Here's how the part is built. I have some questions about the finished solid (model axes, mm). A direction names the side the tool comes from. Round coordinates to 2 decimals unless told otherwise and drop trailing zeros. Write each loop counter-clockwise with the first axis right and the second up, starting at its lowest first coordinate (ties: lowest second). Pieces come first, ordered by that corner, then holes. Notation, with made-up numbers: (34, 25.25) -> (65, 25.25) arc R9 cw to (65, 34.25) -> close; hole circle Ø11 at (-16.75, 64). An arc over 180 degrees is marked (long way). Answer as CSV lines item,"result".
```python
from build123d import *

# Parameters (mm, degrees)
FILLET1_R           = 0.25
SKETCH2_R           = 3
BOSS_EXTRUDE1_DEPTH = 2


with BuildPart() as part:
    # Sketch1 → Revolve1 (revolve)
    with BuildSketch(Plane.XY, mode=Mode.PRIVATE) as revolve1_sk:
        with BuildLine():
            Line((0, 2), (0, 0))
            Line((0, 0), (8.5, 0))
            Line((8.5, 0), (8.5, 4))
            add(Edge.make_bspline(
                [(0, 2), (2.747861556, 2.169330532), (5.476127383, 2.511075109), (8.5, 4)],
                knots=[0, 0, 0, 0, 1, 1, 1, 1], degree=3))
        make_face()
    revolve(revolve1_sk.sketch.rotate(Axis((0, 2, 0), (0, -1, 0)), 180), axis=Axis((0, 2, 0), (0, -1, 0)))

    # Fillet1
    fillet1_edges = [part.edges().sort_by_distance(p)[0] for p in [
        (8.5, 4, 0),
    ]]
    fillet(fillet1_edges, radius=FILLET1_R)

    # Sketch2 → Boss-Extrude1 (add)
    with BuildSketch(Plane.XZ):
        Circle(SKETCH2_R)
    extrude(amount=BOSS_EXTRUDE1_DEPTH)


solid = part.part
```
1. If I drill on line 1 (Y direction, x = -5, z = 4.5); line 2 (Z direction, x = -7, y = 0.95); line 3 (Y direction, x = -0.5, z = 2.5), over which ranges is the centre line in solid material (lowest first)?
Numbers:
line 1,"y = 0 to 3.24"
line 2,"z = -4.82 to 4.82"
line 3,"y = -2 to 2.23"
2. For pin 1 Ø2 at (x, y) = (1, 1.5) entering from -Z; pin 2 Ø1 at (x, z) = (2.5, -2.5) entering from +Y; pin 3 Ø5 at (x, z) = (2, -3.5) entering from +Y; pin 4 Ø1.5 at (y, z) = (-0.5, 1.5) entering from -X, each with a flat end and sliding along its axis, tell me the tip position at first contact or that it passes through.
Numbers:
pin 1,"stops at z = -8.5"
pin 2,"stops at y = 2.48"
pin 3,"stops at y = 3.17"
pin 4,"stops at x = -8.45"
3. Suppose I cut it at B-B on y = 1.8. Please give me the cut outline in (x, z).
Numbers:
outline,"circle Ø17 at (0, 0)"
4. Suppose I cut it at A-A on y = -1.05. Please give me the cut outline in (x, z), and give its area (3 significant figures).
Numbers:
outline,"circle Ø6 at (0, 0)"
area,"28.3 mm^2"
5. On a 3-axis mill with a long thin cutter (end or side, diameter ignored), from which of +Z, -Z, +X, -X, +Y, -Y can I reach the whole of each face in a straight line? I mean faces 1 (the face through (-8.11, 1.83, -2.55)), 2 (the face through (4, 0, 0)). Say none if no direction works.
Numbers:
face 1,"+Y, -Y"
face 2,"-Y"
